Autodesk Inventor part; units mm, degrees
sketch "Sketch2" plane through (0, 0, 0) normal (1, 0, 0) x (0, 1, 0)
  line L0 (50, 25) -> (-50, 25)
  line L1 (-50, 25) -> (-50, -25)
  line L2 (-50, -25) -> (50, -25)
  line L3 (50, -25) -> (50, 25)
  line L4 (-70, 0) -> (70, 0)
  line L5 (0, 35) -> (0, -35)
  line L6 (-50, 25) -> (50, -25)
  point P0 (0, 0)
  point P1 (50, 0)
  point P2 (0, 25)
  dimension "d0" = 50
  dimension "d1" = 100
extrude "Extrusion1" add sketch "Sketch2" along normal mid plane 10 contours L6 L4 L1 | L5 L2 L1 L4 | L6 L2 L5
sketch "Sketch4" plane through (5, 0, 0) normal (1, 0, 0) x (0, 0, -1)
  line L0 (25, 50) -> (-25, -50)
  line L1 (25, -50) -> (25, 50)
  line L2 (-25, -50) -> (25, -50)
  line L3 (22, 37.2918) -> (-20.1459, -47)
  line L4 (-20.1459, -47) -> (22, -47)
  line L5 (22, -47) -> (22, 37.2918)
  point P0 (0, 0)
  dimension "d8" = 3
extrude "Extrusion2" cut sketch "Sketch4" against normal blind 7 contours L5 L4 L3
sketch "Sketch5" plane through (-5, -50, -25) normal (0, -1, 0) x (1, 0, 0)
  line L0 (5, 60) -> (5, -10)
  circle A0 centre (5, 45) radius 2.5
  line L1 (10, 50) -> (0, 50)
  circle A1 centre (5, 5) radius 2.5
  point P0 (5, 25)
  dimension "d11" = 5
  dimension "d12" = 5
  dimension "d15" = 40
extrude "Extrusion3" add sketch "Sketch5" along normal blind 5
sketch "Sketch8" plane through (-5, -50, 25) normal (0, 0.4472, 0.8944) x (1, 0, 0)
  line L0 (10, 0) -> (0, 0)
  line L1 (0, 111.8034) -> (10, 111.8034)
  circle A0 centre (5, 85.9017) radius 2.5
  line L2 (5, 134.1641) -> (5, -22.3607)
  line L3 (-2, 55.9017) -> (12, 55.9017)
  circle A1 centre (5, 25.9017) radius 2.5
  point P0 (5, 55.9017)
  dimension "d31" = 111.8034
  dimension "d32" = 5
  dimension "d34" = 30
extrude "Extrusion4" cut sketch "Sketch8" against normal blind 7
properties part number "Roof_Wall_Large_Left"
Can you work these out from the model? Positions are in its coordinate system, mm. A direction names the side the tool comes from. Coordinates: 2 decimals unless noted, no trailing zeros. Write each loop counter-clockwise with the first axis right and the second up, starting at its lowest first coordinate (ties: lowest second). Pieces come first, ordered by that corner, then holes. Notation, with made-up numbers: (57.25, 30) -> (88.25, 30) arc R17 ccw to (88.25, 53) -> close; hole circle Ø1 at (67.5, -1.75). An arc over 180 degrees is marked (long way). Answer as CSV lines item,"result".
1) If we section it at A-A on x = 0: Please give me the cut outline in (y, z).
Check result:
outline,"(-55, -22.5) -> (-50, -22.5) -> (-50, -25) -> (50, -25) -> (29.07, -14.53) -> (27.73, -17.22) -> (37.29, -22) -> (-47, -22) -> (-47, 20.15) -> (-30.41, 11.85) -> (-29.07, 14.53) -> (-50, 25) -> (-50, 22.5) -> (-55, 22.5) -> (-55, 17.5) -> (-50, 17.5) -> (-50, -17.5) -> (-55, -17.5) -> close; (-25.94, 9.62) -> (23.26, -14.98) -> (24.6, -12.3) -> (-24.6, 12.3) -> close"
2) Will these pins go through, and if not, where does the flat tip stop? P1, Ø12.5, axis at y = -10.5, z = -5.5, coming from the +X side; P2, Ø5.5, axis at x = 1.5, z = -5, coming from the +Y side; P3, Ø1, axis at x = -2.5, z = -18, coming from the +Y side.
Check result:
P1,"x = -2"
P2,"y = 15.5"
P3,"y = 37"
3) On a 3-axis mill with a long thin cutter (end or side, diameter ignored), from which of +Z, -Z, +X, -X, +Y, -Y can I reach the whole of each face in a straight line? I mean faces 5 (the flat face through (2, -5, -22)), 6 (the flat face through (5, -15, -24)), 7 (the cylindrical face through (-0.33, -52.46, -22.48)). Say none if no direction works.
Check result:
face 5,"+X"
face 6,"+Z, -Z, +X, +Y, -Y"
face 7,"-Y"
4) If we section it at B-B on y = 4: Please give me the cut outline in (x, z).
Check result:
outline,"(-5, -25) -> (5, -25) -> (5, -22) -> (-2, -22) -> (-2, -5.35) -> (5, -5.35) -> (5, -2) -> (-5, -2) -> close"
5) If I drill on line 1 (Y direction, x = -1.5, z = 12); line 2 (X direction, y = -24.5, z = -15); line 3 (Y direction, x = -3.5, z = 11), over which ranges is the centre line in solid material (lowest first)? Write a range as from..to.
Check result:
line 1,"-50..-47, -30.71..-29.78, -25.3..-24"
line 2,"-5..-2"
line 3,"-50..-22"
6) If we mould it in two halves opening along Y, with no side actions, what happens to faces 1 (the flat face through (-2, -23, -10)), 2 (the flat face through (2, -47, -1)), 3 (the flat face through (-0.07, -0.7, 0.35)), 4 (the flat face through (0, -55, 20))? For each: +Y half, -Y half, draft (parallel to the pull), parting line (faces both ways), or undercut.
Check result:
face 1,"undercut"
face 2,"undercut"
face 3,"+Y half"
face 4,"-Y half"
7) If we section it at C-C on z = -9: Please give me the cut outline in (x, y).
Check result:
outline,"(-5, -50) -> (5, -50) -> (5, -47) -> (-2, -47) -> (-2, 11.29) -> (5, 11.29) -> (5, 18) -> (-5, 18) -> close"
